Check sheet for the modelled part. Datum: model origin and axes. Units: mm. Round coordinates to 2 decimals unless told otherwise and drop trailing zeros. Loops run counter-clockwise (first coordinate to the right, second up) from the corner with the lowest first, then second, coordinate; pieces in that order, holes last. Notation, with made-up numbers: M 26.25,-9.5 L 64.25,-9.5 A27 ccw 64.25,29.5 Z; hole C -34.5,57 d7. An arc over 180 degrees is marked long. One line per question, with ' | ' between items. Start each with the question number.
(1) Section check D-D (x = -108). Record the boundary of the cut face in (y, z), and give its area (3 significant figures).
(2) Thickness scan on probe 1 along Z at (x, y) = (-207, 23.5); probe 2 along X at (y, z) = (14.5, -286); probe 3 along X at (y, z) = (9, 323). Record the ranges inside material, lowest first. Write a range as [from, to].
(3) Section check A-A (y = 9.5). Count the separate pieces of the cut face and the enclosed holes in it, and give its area (3 significant figures).
(4) Section check B-B (z = 99). Record the boundary of the cut face in (x, y), and give its area (3 significant figures).
(5) Section check C-C (x = 249). Record the boundary of the cut face in (y, z), and give its area (3 significant figures).
```python
from build123d import *

# Parameters (mm, degrees)
SKETCH1_W            = 819
SKETCH1_H            = 819
SKETCH1_W_2          = 759
SKETCH1_H_2          = 759
BOSS_EXTRUDE1_DEPTH  = 3
SKETCH2_W            = 819
SKETCH2_H            = 819
SKETCH2_W_2          = 813
SKETCH2_H_2          = 813
BOSS_EXTRUDE2_DEPTH  = 27
BOSS_EXTRUDE3_DEPTH  = 3
CUT_EXTRUDE1_DEPTH   = 130
BOSS_EXTRUDE4_DEPTH  = 3
BOSS_EXTRUDE5_DEPTH  = 27
CUT_EXTRUDE2_DEPTH   = 163
MIRROR3_DEPTH        = 30
MIRROR3_2_DEPTH      = 3
MIRROR4_DEPTH        = 30
MIRROR4_2_DEPTH      = 3
CUT_EXTRUDE3_START   = -673
CUT_EXTRUDE3_DEPTH   = 1124
CUT_EXTRUDE4_DEPTH   = 300
BOSS_EXTRUDE8_DEPTH  = 3
BOSS_EXTRUDE9_DEPTH  = 27
BOSS_EXTRUDE10_DEPTH = 3
CUT_EXTRUDE9_DEPTH   = 266
CUT_EXTRUDE10_DEPTH  = 27
CUT_EXTRUDE11_DEPTH  = 27
BOSS_EXTRUDE13_DEPTH = 27
BOSS_EXTRUDE15_DEPTH = 3
BOSS_EXTRUDE16_DEPTH = 27
MIRROR17_DEPTH       = 3
MIRROR17_START       = 3
MIRROR17_2_DEPTH     = 27
MIRROR26_DEPTH       = 3
MIRROR26_START       = 3
MIRROR26_2_DEPTH     = 27


# Read off the part's stored shape, not the designer's step: Mirror3, Mirror4, Mirror17, Mirror26
with BuildPart() as part:
    # Sketch1 → Boss-Extrude1 (new body)
    with BuildSketch(Plane(origin=(0, 0, 0), x_dir=(1, 0, 0), z_dir=(0, 1, 0))):
        Rectangle(SKETCH1_W, SKETCH1_H)
        Rectangle(SKETCH1_W_2, SKETCH1_H_2, mode=Mode.SUBTRACT)
    extrude(amount=BOSS_EXTRUDE1_DEPTH)

    # Sketch2 → Boss-Extrude2 (add)
    with BuildSketch(Plane(origin=(0, 3, 0), x_dir=(1, 0, 0), z_dir=(0, 1, 0))):
        Rectangle(SKETCH2_W, SKETCH2_H)
        Rectangle(SKETCH2_W_2, SKETCH2_H_2, mode=Mode.SUBTRACT)
    extrude(amount=BOSS_EXTRUDE2_DEPTH)

    # Sketch3 → Boss-Extrude3 (add)
    with BuildSketch(Plane.XZ):
        Polygon((-294.643593129, 379.5), (-337.07, 379.5), (-379.5, 337.07), (-379.5, 294.643593129), align=None)
    extrude(amount=-BOSS_EXTRUDE3_DEPTH)

    # Sketch4 → Cut-Extrude1 (cut)
    with BuildSketch(Plane(origin=(0, 0, 0), x_dir=(-1, 0, 0), z_dir=(0, -1, 0))):
        Polygon((358.285, -358.285), (409.5, -307.07), (409.5, -409.5), (307.07, -409.5), align=None)
    extrude(amount=-CUT_EXTRUDE1_DEPTH, mode=Mode.SUBTRACT)

    # Sketch7 → Boss-Extrude4 (add)
    with BuildSketch(Plane(origin=(0, 0, 0), x_dir=(-1, 0, 0), z_dir=(0, -1, 0))):
        Polygon((409.5, -109.080101268), (409.5, -73.724762208), (73.724762208, -409.5), (109.080101268, -409.5), align=None)
    extrude(amount=-BOSS_EXTRUDE4_DEPTH)

    # Sketch8 → Boss-Extrude5 (add)
    with BuildSketch(Plane(origin=(0, 3, 0), x_dir=(1, 0, 0), z_dir=(0, 1, 0))):
        Polygon((-406.5, -76.724762208), (-406.5, -80.967402896), (-80.967402896, -406.5), (-76.724762208, -406.5), align=None)
    extrude(amount=BOSS_EXTRUDE5_DEPTH)

    # Sketch10 → Cut-Extrude2 (cut)
    with BuildSketch(Plane(origin=(0, 0, 0), x_dir=(-1, 0, 0), z_dir=(0, -1, 0))):
        Polygon((0, -409.5), (0, 0), (409.5, 0), (409.5, 409.5), (-409.5, 409.5), (-409.5, -409.5), align=None)
    extrude(amount=-CUT_EXTRUDE2_DEPTH, mode=Mode.SUBTRACT)

    # Mirror3 outline → Mirror3 (add)
    with BuildSketch(Plane(origin=(0, 0, 0), x_dir=(1, 0, 0), z_dir=(0, 1, 0))):
        Polygon((406.5, -76.724762208), (76.724762208, -406.5), (0, -406.5), (0, -409.5), (307.07, -409.5), (310.07, -406.5), (80.967402896, -406.5), (406.5, -80.967402896), (406.5, -310.07), (409.5, -307.07), (409.5, 0), (406.5, 0), align=None)
    extrude(amount=MIRROR3_DEPTH)

    # Mirror3 2 outline → Mirror3 2 (add)
    # profile 1 of 3: a face of its own
    with BuildSketch(Plane(origin=(0, 0, 0), x_dir=(1, 0, 0), z_dir=(0, 1, 0))):
        Polygon((0, -406.5), (76.724762208, -406.5), (103.724762208, -379.5), (0, -379.5), align=None)
    # profile 2 of 3: a face of its own
    with BuildSketch(Plane(origin=(0, 0, 0), x_dir=(1, 0, 0), z_dir=(0, 1, 0))):
        Polygon((379.5, 0), (379.5, -103.724762208), (406.5, -76.724762208), (406.5, 0), align=None)
    # profile 3 of 3: a face of its own
    with BuildSketch(Plane(origin=(0, 0, 0), x_dir=(1, 0, 0), z_dir=(0, 1, 0))):
        Polygon((80.967402896, -406.5), (310.07, -406.5), (406.5, -310.07), (406.5, -80.967402896), align=None)
        Polygon((379.5, -294.643593129), (294.643593129, -379.5), (139.080101268, -379.5), (379.5, -139.080101268), align=None, mode=Mode.SUBTRACT)
    extrude(amount=MIRROR3_2_DEPTH)

    # Mirror4 outline → Mirror4 (add)
    with BuildSketch(Plane(origin=(0, 0, 0), x_dir=(1, 0, 0), z_dir=(0, 1, 0))):
        Polygon((-409.5, 0), (-406.5, 0), (-406.5, 76.724762208), (-76.724762208, 406.5), (76.724762208, 406.5), (406.5, 76.724762208), (406.5, 0), (409.5, 0), (409.5, 307.07), (406.5, 310.07), (406.5, 80.967402896), (80.967402896, 406.5), (310.07, 406.5), (307.07, 409.5), (-307.07, 409.5), (-310.07, 406.5), (-80.967402896, 406.5), (-406.5, 80.967402896), (-406.5, 310.07), (-409.5, 307.07), align=None)
    extrude(amount=MIRROR4_DEPTH)

    # Mirror4 2 outline → Mirror4 2 (add)
    # profile 1 of 5: a face of its own
    with BuildSketch(Plane(origin=(0, 0, 0), x_dir=(1, 0, 0), z_dir=(0, 1, 0))):
        Polygon((-406.5, 76.724762208), (-406.5, 0), (-379.5, 0), (-379.5, 103.724762208), align=None)
    # profile 2 of 5: a face of its own
    with BuildSketch(Plane(origin=(0, 0, 0), x_dir=(1, 0, 0), z_dir=(0, 1, 0))):
        Polygon((-76.724762208, 406.5), (-103.724762208, 379.5), (103.724762208, 379.5), (76.724762208, 406.5), align=None)
    # profile 3 of 5: a face of its own
    with BuildSketch(Plane(origin=(0, 0, 0), x_dir=(1, 0, 0), z_dir=(0, 1, 0))):
        Polygon((-310.07, 406.5), (-406.5, 310.07), (-406.5, 80.967402896), (-80.967402896, 406.5), align=None)
        Polygon((-139.080101268, 379.5), (-379.5, 139.080101268), (-379.5, 294.643593129), (-294.643593129, 379.5), align=None, mode=Mode.SUBTRACT)
    # profile 4 of 5: a face of its own
    with BuildSketch(Plane(origin=(0, 0, 0), x_dir=(1, 0, 0), z_dir=(0, 1, 0))):
        Polygon((406.5, 76.724762208), (379.5, 103.724762208), (379.5, 0), (406.5, 0), align=None)
    # profile 5 of 5: a face of its own
    with BuildSketch(Plane(origin=(0, 0, 0), x_dir=(1, 0, 0), z_dir=(0, 1, 0))):
        Polygon((406.5, 310.07), (310.07, 406.5), (80.967402896, 406.5), (406.5, 80.967402896), align=None)
        Polygon((294.643593129, 379.5), (379.5, 294.643593129), (379.5, 139.080101268), (139.080101268, 379.5), align=None, mode=Mode.SUBTRACT)
    extrude(amount=MIRROR4_2_DEPTH)

    # Sketch12 → Cut-Extrude3 (cut)
    with BuildSketch(Plane(origin=(0, 0, 0), x_dir=(-1, 0, 0), z_dir=(0, -1, 0)).offset(CUT_EXTRUDE3_START)):
        Polygon((379.5, -337.07), (379.5, -294.643593129), (294.643593129, -379.5), (337.07, -379.5), align=None)
    extrude(amount=CUT_EXTRUDE3_DEPTH, mode=Mode.SUBTRACT)

    # Sketch13 → Cut-Extrude4 (cut)
    with BuildSketch(Plane.XZ):
        Polygon((-409.5, 0), (0, 0), (0, 409.5), (505.643397908, 433.197413997), (586.960318624, -390.321219438), (40.755373804, -460.11749056), (-470.159650687, -449.460798141), align=None)
    extrude(amount=-CUT_EXTRUDE4_DEPTH, mode=Mode.SUBTRACT)

    # Sketch14 → Boss-Extrude8 (add)
    with BuildSketch(Plane.XZ):
        Polygon((-409.5, 307.07), (-307.07, 409.5), (-335.354271247, 409.5), (-409.5, 335.354271247), align=None)
    extrude(amount=-BOSS_EXTRUDE8_DEPTH)

    # Sketch16 → Boss-Extrude9 (add)
    with BuildSketch(Plane(origin=(0, 3, 0), x_dir=(1, 0, 0), z_dir=(0, 1, 0))):
        Polygon((-409.5, -307.07), (-406.5, -310.07), (-406.5, -338.354271247), (-409.5, -335.354271247), align=None)
        Polygon((-307.07, -409.5), (-310.07, -406.5), (-338.354271247, -406.5), (-335.354271247, -409.5), align=None)
    extrude(amount=BOSS_EXTRUDE9_DEPTH)

    # Sketch17 → Boss-Extrude10 (add)
    with BuildSketch(Plane(origin=(0, 0, 0), x_dir=(-1, 0, 0), z_dir=(0, -1, 0))):
        Polygon((181.506508139, -379.5), (379.5, -181.506508139), (379.5, -139.080101268), (139.080101268, -379.5), align=None)
    extrude(amount=-BOSS_EXTRUDE10_DEPTH)

    # Sketch18 → Cut-Extrude9 (cut)
    with BuildSketch(Plane(origin=(0, 0, 0), x_dir=(-1, 0, 0), z_dir=(0, -1, 0))):
        Polygon((379.5, -103.724762208), (103.724762208, -379.5), (139.080101268, -379.5), (379.5, -139.080101268), align=None)
    extrude(amount=-CUT_EXTRUDE9_DEPTH, mode=Mode.SUBTRACT)

    # Sketch19 → Cut-Extrude10 (cut)
    with BuildSketch(Plane(origin=(0, 30, 0), x_dir=(1, 0, 0), z_dir=(0, 1, 0))):
        Polygon((-406.5, -80.967402896), (-406.5, -76.724762208), (-379.5, -103.724762208), (-379.5, -107.967402896), align=None)
    extrude(amount=-CUT_EXTRUDE10_DEPTH, mode=Mode.SUBTRACT)

    # Sketch20 → Cut-Extrude11 (cut)
    with BuildSketch(Plane(origin=(0, 30, 0), x_dir=(1, 0, 0), z_dir=(0, 1, 0))):
        Polygon((-107.967402896, -379.5), (-103.724762208, -379.5), (-76.724762208, -406.5), (-80.967402896, -406.5), align=None)
    extrude(amount=-CUT_EXTRUDE11_DEPTH, mode=Mode.SUBTRACT)

    # Sketch21 → Boss-Extrude13 (add)
    with BuildSketch(Plane(origin=(0, 3, 0), x_dir=(1, 0, 0), z_dir=(0, 1, 0))):
        Polygon((-379.5, -181.506508139), (-181.506508139, -379.5), (-177.263867452, -379.5), (-379.5, -177.263867452), align=None)
    extrude(amount=BOSS_EXTRUDE13_DEPTH)

    # Sketch22 → Boss-Extrude15 (add)
    with BuildSketch(Plane(origin=(0, 0, 0), x_dir=(-1, 0, 0), z_dir=(0, -1, 0))):
        Polygon((409.5, -335.354271247), (335.354271247, -409.5), (349.496406871, -409.5), (409.5, -349.496406871), align=None)
    extrude(amount=-BOSS_EXTRUDE15_DEPTH)

    # Sketch23 → Boss-Extrude16 (add)
    with BuildSketch(Plane(origin=(0, 3, 0), x_dir=(1, 0, 0), z_dir=(0, 1, 0))):
        Polygon((-406.5, -338.354271247), (-409.5, -335.354271247), (-409.5, -349.496406871), (-406.5, -352.496406871), align=None)
        Polygon((-338.354271247, -406.5), (-352.496406871, -406.5), (-349.496406871, -409.5), (-335.354271247, -409.5), align=None)
    extrude(amount=BOSS_EXTRUDE16_DEPTH)

    # Mirror17 outline → Mirror17 (add)
    with BuildSketch(Plane(origin=(0, 0, 0), x_dir=(1, 0, 0), z_dir=(0, 1, 0))):
        Polygon((379.5, -139.080101268), (139.080101268, -379.5), (0, -379.5), (0, -409.5), (349.496406871, -409.5), (409.5, -349.496406871), (409.5, 0), (379.5, 0), align=None)
        Polygon((379.5, -337.07), (337.07, -379.5), (181.506508139, -379.5), (379.5, -181.506508139), align=None, mode=Mode.SUBTRACT)
    extrude(amount=MIRROR17_DEPTH)

    # Mirror17 2 outline → Mirror17 2 (add)
    with BuildSketch(Plane(origin=(0, 0, 0), x_dir=(1, 0, 0), z_dir=(0, 1, 0)).offset(MIRROR17_START)):
        Polygon((352.496406871, -406.5), (0, -406.5), (0, -409.5), (349.496406871, -409.5), align=None)
        Polygon((409.5, 0), (406.5, 0), (406.5, -352.496406871), (409.5, -349.496406871), align=None)
        Polygon((177.263867452, -379.5), (181.506508139, -379.5), (379.5, -181.506508139), (379.5, -177.263867452), align=None)
    extrude(amount=MIRROR17_2_DEPTH)

    # Mirror26 outline → Mirror26 (add)
    with BuildSketch(Plane(origin=(0, 0, 0), x_dir=(1, 0, 0), z_dir=(0, 1, 0))):
        Polygon((-379.5, 0), (-379.5, 139.080101268), (-139.080101268, 379.5), (139.080101268, 379.5), (379.5, 139.080101268), (379.5, 0), (409.5, 0), (409.5, 349.496406871), (349.496406871, 409.5), (-349.496406871, 409.5), (-409.5, 349.496406871), (-409.5, 0), align=None)
        Polygon((-337.07, 379.5), (-181.506508139, 379.5), (-379.5, 181.506508139), (-379.5, 337.07), align=None, mode=Mode.SUBTRACT)
        Polygon((337.07, 379.5), (379.5, 337.07), (379.5, 181.506508139), (181.506508139, 379.5), align=None, mode=Mode.SUBTRACT)
    extrude(amount=MIRROR26_DEPTH)

    # Mirror26 2 outline → Mirror26 2 (add)
    with BuildSketch(Plane(origin=(0, 0, 0), x_dir=(1, 0, 0), z_dir=(0, 1, 0)).offset(MIRROR26_START)):
        Polygon((-409.5, 0), (-406.5, 0), (-406.5, 352.496406871), (-409.5, 349.496406871), align=None)
        Polygon((-349.496406871, 409.5), (-352.496406871, 406.5), (352.496406871, 406.5), (349.496406871, 409.5), align=None)
        Polygon((409.5, 349.496406871), (406.5, 352.496406871), (406.5, 0), (409.5, 0), align=None)
        Polygon((-181.506508139, 379.5), (-379.5, 181.506508139), (-379.5, 177.263867452), (-177.263867452, 379.5), align=None)
        Polygon((379.5, 177.263867452), (379.5, 181.506508139), (181.506508139, 379.5), (177.263867452, 379.5), align=None)
    extrude(amount=MIRROR26_2_DEPTH)


solid = part.part
```
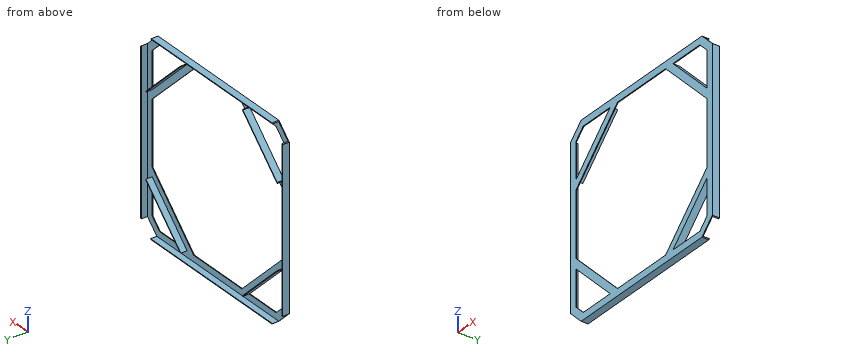
The answers:
1) outline: M 0,-409.5 L 30,-409.5 L 30,-406.5 L 3,-406.5 L 3,-379.5 L 0,-379.5 Z; M 0,379.5 L 3,379.5 L 3,406.5 L 30,406.5 L 30,409.5 L 0,409.5 Z | area: 342 mm²
2) probe 1: [-409.5, -406.5], [-354.01, -349.76], [349.76, 354.01], [406.5, 409.5] | probe 2: [-409.5, -406.5], [-275.01, -270.76], [270.76, 275.01], [406.5, 409.5] | probe 3: [-409.5, -406.5], [-238.01, -233.76], [233.76, 238.01], [406.5, 409.5]
3) separate pieces: 8 | enclosed holes: 0 | area: 11,800 mm²
4) outline: M -409.5,0 L -379.5,0 L -379.5,3 L -406.5,3 L -406.5,30 L -409.5,30 Z; M 379.5,0 L 409.5,0 L 409.5,30 L 406.5,30 L 406.5,3 L 379.5,3 Z | area: 342 mm²
5) outline: M 0,-409.5 L 30,-409.5 L 30,-406.5 L 3,-406.5 L 3,-379.5 L 0,-379.5 Z; M 0,-312.01 L 30,-312.01 L 30,-307.76 L 3,-307.76 L 3,-269.58 L 0,-269.58 Z; M 0,269.58 L 3,269.58 L 3,307.76 L 30,307.76 L 30,312.01 L 0,312.01 Z; M 0,379.5 L 3,379.5 L 3,406.5 L 30,406.5 L 30,409.5 L 0,409.5 Z | area: 826 mm²
